For this review, use the dimensioned drawing (mm, ordinates from the lowest corner) and the shaded views. A direction names the side the tool comes from. Coordinates: 2 decimals unless noted, no trailing zeros. Loops run counter-clockwise (first coordinate to the right, second up) from the corner with the lowest first, then second, coordinate; pieces in that order, holes last. Notation, with made-up numbers: M -22,-8 L 7,-8 A12 ccw 7,6 Z; hole C -28,3 d5. An arc over 180 degrees is marked long. Write item = value, one per line. Start each with the question number.
Q1. We need section D-D on y = 12.5. Give the boundary of the cut face in (x, z).
Q2. For the marked faces 1, 2, 3, 4 and 5, list the 3-axis set-ups (+Z, -Z, +X, -X, +Y, -Y) from which the entire face can be reached by the end or side of a thin tool; tool diameter is ignored.
Q3. We need section A-A on y = 3. Give the boundary of the cut face in (x, z), and give its area (3 significant figures).
Q4. Mouldability with a two-part tool opening along Y and no side actions: class the marked faces 6, 7 and 8 as released by +Y, released by -Y, zero draft, split by the parting line, or undercut.
Q5. Wall thickness on probe 1 along X at (y, z) = (3, 12.6); probe 2 along Z at (x, y) = (3.5, 1); probe 3 along Y at (x, z) = (6.75, 6.25): over which ranges is each line inside the solid? List them lowest first.
Q6. We need section B-B on z = 9. Give the boundary of the cut face in (x, y).
Q7. We need section C-C on x = 4. Count the separate pieces of the cut face and the enclosed holes in it.
Q8. Clearance check with flat-ended pins moving along their axes: pin 1 Ø1.8 at (x, y) = (4, 26.5) entering from +Z; pin 2 Ø3 at (y, z) = (10, 5) entering from +X; pin 3 Ø1.8 at (x, y) = (5.5, 26.5) entering from -Z; pin 4 Ø2 at (x, y) = (4, 3) entering from +Z. State where each tip first meets the part, or that it passes through.
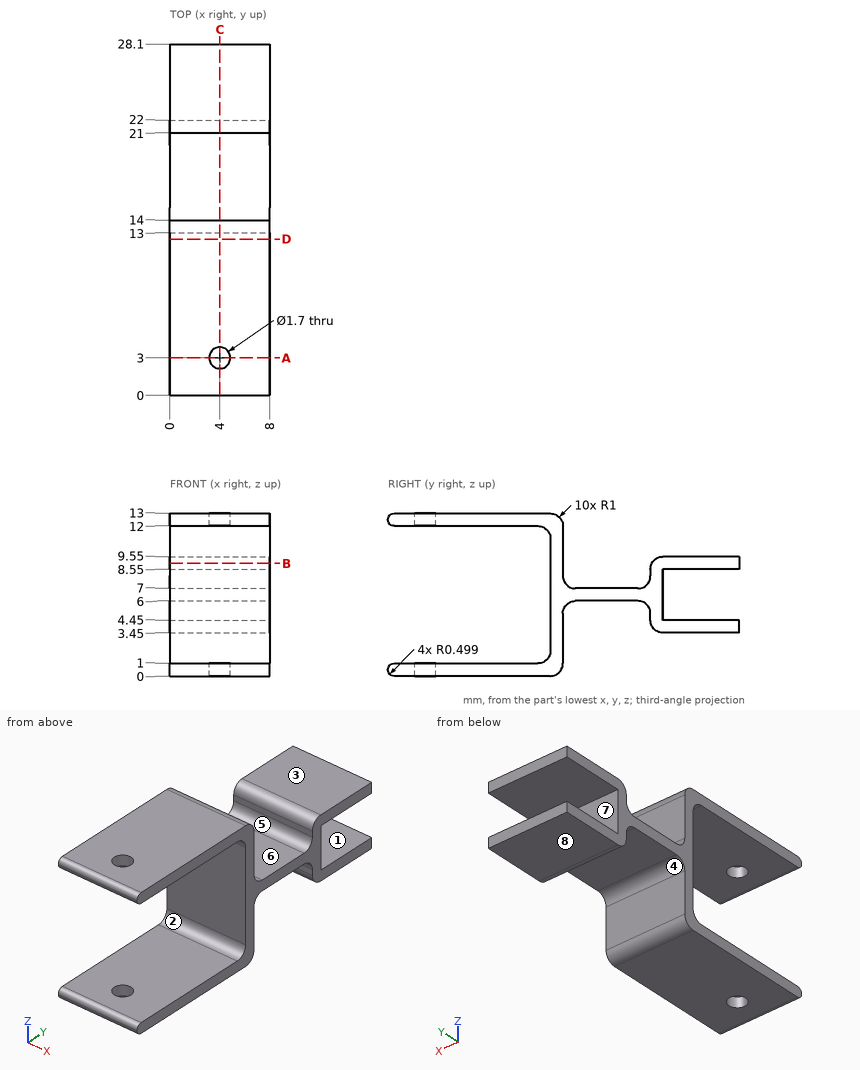
Returned:
q1.outline = M 0,0 L 8,0 L 8,1.13 L 0,1.13 Z; M 0,11.87 L 8,11.87 L 8,13 L 0,13 Z
q2.face_1 = +X, -X, +Y
q2.face_2 = +X, -X, -Y
q2.face_3 = +Z, +X, -X, +Y
q2.face_4 = -Z, +X, -X
q2.face_5 = +Z, +X, -X
q3.outline = M 0,0 L 3.15,0 L 3.15,1 L 0,1 Z; M 0,12 L 3.15,12 L 3.15,13 L 0,13 Z; M 4.85,0 L 8,0 L 8,1 L 4.85,1 Z; M 4.85,12 L 8,12 L 8,13 L 4.85,13 Z
q3.area = 12.6 mm^2
q4.face_6 = undercut
q4.face_7 = released by +Y
q4.face_8 = zero draft
q5.probe_1 = 0 to 3.15, 4.85 to 8
q5.probe_2 = 0 to 1, 12 to 13
q5.probe_3 = 13 to 22
q6.outline = M 0,13 L 8,13 L 8,14 L 0,14 Z; M 0,21.11 L 8,21.11 L 8,28.1 L 0,28.1 Z
q7.separate_pieces = 3
q7.enclosed_holes = 0
q8.pin_1 = 9.55
q8.pin_2 = through
q8.pin_3 = 3.45
q8.pin_4 = 13
